from build123d import *

# Parameters (mm, degrees)
SKETCH_1_R             = 7
SM_BASE_FLANGE_1_DEPTH = 4


# Sheet-metal steps are written as plain solids
with BuildPart() as part:
    # Sketch 1 → Базовая кромка1 (new body)
    with BuildSketch(Plane(origin=(0, 0, 0), x_dir=(0, 0, -1), z_dir=(1, 0, 0))):
        with BuildLine():
            Line((0, 20), (235, 20))
            ThreePointArc((235, 20), (255, 0), (235, -20))
            Line((235, -20), (0, -20))
            ThreePointArc((0, -20), (-20, 0), (0, 20))
        make_face()
        Circle(SKETCH_1_R, mode=Mode.SUBTRACT)
        with Locations((235, 0)):
            Circle(SKETCH_1_R, mode=Mode.SUBTRACT)
    extrude(amount=-SM_BASE_FLANGE_1_DEPTH)


solid = part.part
Geometry check sheet. Reference: the model listing, model coordinates, mm. Round coordinates to 2 decimals unless told otherwise and drop trailing zeros. Loops run counter-clockwise (first coordinate to the right, second up) from the corner with the lowest first, then second, coordinate; pieces in that order, holes last. Notation, with made-up numbers: (62, 67.25) -> (70, 67.25) arc R22 cw to (70, 91.25) -> close; hole circle Ø8 at (75.25, -35). An arc over 180 degrees is marked (long way). Answer as a JSON object with one key per item and string values. Group by question number.
Item 1: Cross-section at A-A, the plane x = -1.5. Record the cut outline in (y, z), plus the area to 3 significant figures.
Item 2: Cross-section at B-B, the plane y = 0. Record the cut outline in (x, z).
Item 3: Depth check by flat-ended pin: pin 1 Ø3 at (y, z) = (11.5, -30) entering from +X; pin 2 Ø11 at (y, z) = (0, 0) entering from +X. Enter the tip coordinate at first touch or a pass-through.
Item 4: Release check for a two-part mould opening along Y. For faces 1 (the face through (-1.972, -2.681, -6.466)), 2 (the face through (-4, 0, -119)), 3 (the face through (-2, 0, 20)) record: pulls with the +Y half, pulls with the -Y half, needs draft (parallel to the pull), parting line crosses it, or undercut.
Item 5: Thickness scan on line 1 along Z through (x, y) = (-1.25, 1.5); line 2 along Y through (x, z) = (-1.65, -235); line 3 along Y through (x, z) = (-1.85, -241). Record the ranges inside material, lowest first.
Item 6: Cross-section at C-C, the plane y = 10. Record the cut outline in (x, z), plus the area to 3 significant figures.
Determined:
{
 "1": {"outline": "(-20, -235) arc R20 ccw to (20, -235) -> (20, 0) arc R20 ccw to (-20, 0) -> close; hole circle Ø14 at (0, -235); hole circle Ø14 at (0, 0)", "area": "10,300 mm²"},
 "2": {"outline": "(-4, -255) -> (0, -255) -> (0, -242) -> (-4, -242) -> close; (-4, -228) -> (0, -228) -> (0, -7) -> (-4, -7) -> close; (-4, 7) -> (0, 7) -> (0, 20) -> (-4, 20) -> close"},
 "3": {"pin 1": "stops at x = 0", "pin 2": "passes through"},
 "4": {"face 1": "undercut", "face 2": "needs draft", "face 3": "parting line crosses it"},
 "5": {"line 1": "z = -254.94 to -241.84, -228.16 to -6.84, 6.84 to 19.94", "line 2": "y = -20 to -7, 7 to 20", "line 3": "y = -19.08 to -3.61, 3.61 to 19.08"},
 "6": {"outline": "(-4, -252.32) -> (0, -252.32) -> (0, 17.32) -> (-4, 17.32) -> close", "area": "1,080 mm²"}
}
